```python
from build123d import *

# Parameters (mm, degrees)
SKETCH1_W           = 110
SKETCH1_H           = 110
BOSS_EXTRUDE1_DEPTH = 15
SKETCH3_R           = 4.25
CUT_EXTRUDE1_DEPTH  = 15
FILLET1_R           = 10
SKETCH4_R           = 40
BOSS_EXTRUDE2_DEPTH = 80


with BuildPart() as part:
    # Sketch1 → Boss-Extrude1 (new body)
    with BuildSketch(Plane(origin=(0, 0, 0), x_dir=(1, 0, 0), z_dir=(0, 1, 0))):
        with Locations((11.233421751, -25.384615385)):
            Rectangle(SKETCH1_W, SKETCH1_H)
    extrude(amount=BOSS_EXTRUDE1_DEPTH)

    # Sketch3 → Cut-Extrude1 (cut)
    with BuildSketch(Plane(origin=(0, 0, 0), x_dir=(-1, 0, 0), z_dir=(0, -1, 0))):
        with Locations(Location((28.766578249, -65.384615385, 0), (0, 0, 90))):
            Circle(SKETCH3_R)
        with Locations(Location((-51.233421751, -65.384615385, 0), (0, 0, 90))):
            Circle(SKETCH3_R)
        with Locations(Location((-51.233421751, 14.615384615, 0), (0, 0, 90))):
            Circle(SKETCH3_R)
        with Locations(Location((28.766578249, 14.615384615, 0), (0, 0, 90))):
            Circle(SKETCH3_R)
    extrude(amount=-CUT_EXTRUDE1_DEPTH, mode=Mode.SUBTRACT)

    # Fillet1
    fillet1_edges = [part.edges().sort_by_distance(p)[0] for p in [
        (-43.766578249, 7.5, -29.615384615),
        (66.233421751, 7.5, -29.615384615),
        (66.233421751, 7.5, 80.384615385),
        (-43.766578249, 7.5, 80.384615385),
    ]]
    fillet(fillet1_edges, radius=FILLET1_R)

    # Sketch4 → Boss-Extrude2 (add)
    with BuildSketch(Plane(origin=(0, 15, 0), x_dir=(1, 0, 0), z_dir=(0, 1, 0))):
        with Locations(Location((11.233421751, -25.384615385, 0), (0, 0, 270))):
            Circle(SKETCH4_R)
    extrude(amount=BOSS_EXTRUDE2_DEPTH)


solid = part.part
```
Check sheet for the modelled part. Datum: model origin and axes. Units: mm. A direction names the side the tool comes from. Round coordinates to 2 decimals unless told otherwise and drop trailing zeros. Order: outer loops, then holes, each group sorted by start corner. A loop starts at its lowest first (then second) coordinate and runs counter-clockwise, first axis right, second up. Notation, with made-up numbers: M 23,-29 L 59,-29 A10 ccw 59,-25 Z; hole C 0.5,71 d8. An arc over 180 degrees is marked long. Answer in a Markdown table with one row per item.
(1) Section check A-A on x = -26. Record the boundary of the cut face in (y, z), plus the area to 3 significant figures.
Findings:
| item | result |
|---|---|
| outline | M 0,-29.62 L 15,-29.62 L 15,-17.84 L 0,-17.84 Z; M 0,-11.39 L 15,-11.39 L 15,10.77 L 95,10.77 L 95,40 L 15,40 L 15,62.16 L 0,62.16 Z; M 0,68.61 L 15,68.61 L 15,80.38 L 0,80.38 Z |
| area | 3,800 mm^2 |
(2) Material ranges on line 1 along Y through (x, z) = (60, 8); line 2 along X through (y, z) = (90, 26.5); line 3 along X through (y, z) = (69.5, 4), recorded low to high. Write a range as from..to.
Findings:
| item | result |
|---|---|
| line 1 | y = 0..15 |
| line 2 | x = -28.75..51.22 |
| line 3 | x = -22.57..45.04 |
(3) Set-up check for faces 1 (the flat face through (-43.767, 7, 26)), 2 (the cylindrical face through (-27.815, 54.44, 16.713)): record each of +Z, -Z, +X, -X, +Y, -Y from which the full face is reachable in a straight line by a thin tool's end or side.
Findings:
| item | result |
|---|---|
| face 1 | +Z, -Z, -X, +Y, -Y |
| face 2 | +Y |
(4) Gauge pin test, flat ends, axial feed: pin 1 (11 mm diameter, centred on x = 51.23, z = -14.62, fed in from +Y); pin 2 (12 mm diameter, centred on x = 34, y = 64, fed in from +Z); pin 3 (4 mm diameter, centred on y = 27, z = 9, fed in from -X). Record the tip position at first contact, or that the pin passes through.
Findings:
| item | result |
|---|---|
| pin 1 | stops at y = 15 |
| pin 2 | stops at z = 61.7 |
| pin 3 | stops at x = -26.09 |
(5) Section check B-B on z = 28.5. Record the boundary of the cut face in (x, y), plus the area to 3 significant figures.
Findings:
| item | result |
|---|---|
| outline | M -43.77,0 L 66.23,0 L 66.23,15 L 51.11,15 L 51.11,95 L -28.65,95 L -28.65,15 L -43.77,15 Z |
| area | 8,030 mm^2 |
(6) Section check D-D on y = 38. Record the boundary of the cut face in (x, z).
Findings:
| item | result |
|---|---|
| outline | C 11.23,25.38 d80 |
(7) Draft check along Z on faces 3 (the flat face through (11, 7, -29.615)), 4 (the cylindrical face through (-27.49, 7.4, 61.33)), 5 (the cylindrical face through (-24.553, 7.395, -14.062)), 6 (the cylindrical face through (-40.91, 7.6, 77.38)). Enter one of: +Z half, -Z half, draft (parallel to the pull), parting line (faces both ways), or undercut.
Findings:
| item | result |
|---|---|
| face 3 | -Z half |
| face 4 | undercut |
| face 5 | undercut |
| face 6 | +Z half |
(8) Section check C-C on x = 17. Record the boundary of the cut face in (y, z), plus the area to 3 significant figures.
Findings:
| item | result |
|---|---|
| outline | M 0,-29.62 L 15,-29.62 L 15,-14.2 L 95,-14.2 L 95,64.97 L 15,64.97 L 15,80.38 L 0,80.38 Z |
| area | 7,980 mm^2 |
